Geometry check sheet. Reference: the model listing, model coordinates, mm. A direction names the side the tool comes from. Give positions to 0.01 mm unless a question says otherwise; leave off trailing zeros. Loops run counter-clockwise (first coordinate to the right, second up) from the corner with the lowest first, then second, coordinate; pieces in that order, holes last. Notation, with made-up numbers: (77.5, -30) - (122.5, -30) arc R25 cw to (122.5, -18) - close; hole circle Ø9 at (47.5, 69.5). An arc over 180 degrees is marked (long way). Use a Markdown table: item, result. Add a question column.
1. Material ranges on L1, parallel to Z at x = 30, y = 31.5; L2, parallel to Z at x = 22, y = 22.5; L3, parallel to X at y = 42.5, z = 67, recorded low to high.
2. Cross-section at C-C on z = 54. Enter the section's corners in (x, y), and give its area (3 significant figures).
3. Cross-section at A-A on y = 44.5. Enter the section's corners in (x, z), and give its area (3 significant figures).
4. Draft check along Z on faces 1 (the flat face through (-3, 0, -2)), 2 (the flat face through (-3, 30, 175)), 3 (the flat face through (4, 35, 145.831)). Enter one of: pulls with the +Z half, pulls with the -Z half, needs draft (parallel to the pull), parting line crosses it, or undercut.
5. Set-up check for faces 4 (the flat face through (6, 19, 155)), 5 (the flat face through (3, 25, -175)), 6 (the flat face through (-199.159, 35, 7)): record each of +Z, -Z, +X, -X, +Y, -Y from which the full face is reachable in a straight line by a thin tool's end or side.
6. Depth check by flat-ended pin: P1, Ø6, axis at x = 141.5, z = 70, coming from the +Y side; P2, Ø10, axis at x = 13.5, y = 18, coming from the +Z side. Enter the tip coordinate at first touch or a pass-through.
7. Cross-section at B-B on x = 134. Enter the section's corners in (y, z).
from build123d import *

# Parameters (mm, degrees)
SKETCH1_W           = 500
SKETCH1_H           = 350
BOSS_EXTRUDE1_DEPTH = 20
SKETCH2_W           = 412.975976351
SKETCH2_H           = 281.551553033
BOSS_EXTRUDE2_DEPTH = 30
SKETCH3_W           = 87.5
SKETCH3_H           = 12.5
CUT_EXTRUDE2_DEPTH  = 20


with BuildPart() as part:
    # Sketch1 → Boss-Extrude1 (new body)
    with BuildSketch(Plane(origin=(0, 0, 0), x_dir=(1, 0, 0), z_dir=(0, 1, 0))):
        Rectangle(SKETCH1_W, SKETCH1_H)
    extrude(amount=BOSS_EXTRUDE1_DEPTH)

    # Sketch2 → Boss-Extrude2 (add)
    with BuildSketch(Plane(origin=(0, 20, 0), x_dir=(1, 0, 0), z_dir=(0, 1, 0))):
        Polygon((-250, 175), (-199.158549183, 175), (250, 175), (250, 135.720991004), (250, -175), (213.817427168, -175), (-199.158549183, -175), (-250, -175), align=None)
        with Locations((7.329438993, -5.054785513)):
            Rectangle(SKETCH2_W, SKETCH2_H, mode=Mode.SUBTRACT)
    extrude(amount=BOSS_EXTRUDE2_DEPTH)

    # Sketch3 → Cut-Extrude2 (cut)
    with BuildSketch(Plane.XY.offset(175)):
        with Locations((6.25, 18.75)):
            Rectangle(SKETCH3_W, SKETCH3_H)
    extrude(amount=-CUT_EXTRUDE2_DEPTH, mode=Mode.SUBTRACT)


solid = part.part
Values found:
| question | item | result |
|---|---|---|
| 1 | L1 | z = -175 to -135.72, 145.83 to 175 |
| 1 | L2 | z = -175 to -135.72, 145.83 to 155 |
| 1 | L3 | x = -250 to -199.16, 213.82 to 250 |
| 2 | outline | (-250, 0) - (250, 0) - (250, 50) - (213.82, 50) - (213.82, 20) - (-199.16, 20) - (-199.16, 50) - (-250, 50) - close |
| 2 | area | 12,600 mm2 |
| 3 | outline | (-250, -175) - (250, -175) - (250, 175) - (-250, 175) - close; hole (-199.16, -135.72) - (213.82, -135.72) - (213.82, 145.83) - (-199.16, 145.83) - close |
| 3 | area | 58,700 mm2 |
| 4 | face 1 | needs draft |
| 4 | face 2 | pulls with the +Z half |
| 4 | face 3 | undercut |
| 5 | face 4 | +Z |
| 5 | face 5 | -Z, +X, -X, +Y, -Y |
| 5 | face 6 | +Y |
| 6 | P1 | stops at y = 20 |
| 6 | P2 | stops at z = 155 |
| 7 | outline | (0, -175) - (50, -175) - (50, -135.72) - (20, -135.72) - (20, 145.83) - (50, 145.83) - (50, 175) - (0, 175) - close |
